Can you work these out from the model? Positions are in its coordinate system, mm. Face numbers are marked on the shaded views. A direction names the side the tool comes from. Give positions to 0.01 mm unless a question says otherwise; leave off trailing zeros. Order: outer loops, then holes, each group sorted by start corner. A loop starts at its lowest first (then second) coordinate and runs counter-clockwise, first axis right, second up.
Item 1: If I drill on line 1 along X through (y, z) = (15.75, 0); line 2 along Z through (x, y) = (-0.5, 4.5); line 3 along X through (y, z) = (9.5, -31), over which ranges is the centre line in solid material (lowest first)?
Item 2: Which directions (+Z, -Z, +X, -X, +Y, -Y) give clear straight access to the entire face, cutting with the end or side of a thin tool? Please do the marked faces 1, 2 and 3.
Item 3: I want a section at A-A, the plane x = 36. Write out the boundary of the cut face in (y, z).
Item 4: I want a section at B-B, the plane z = -36. Write out the boundary of the cut face in (x, y), then the cut area to 3 significant figures.
Item 5: I'm going to push flat-ended pins straight in: pin 1 Ø16 at (x, z) = (0, -11) entering from -Y; pin 2 Ø9 at (x, z) = (11, 0) entering from +Y; pin 3 Ø1.5 at (x, z) = (-8, 30) entering from -Y; pin 4 Ø4 at (y, z) = (2, -4) entering from -X. Where does each tip first touch, or does it pass through?
Item 6: If we mould it in two halves opening along X, with no side actions, what happens to the marked faces 4, 5 and 6? For each: +X half, -X half, draft (parallel to the pull), parting line (faces both ways), or undercut.
Item 7: I want a section at D-D, the plane z = 31. Write out the boundary of the cut face in (x, y).
Item 8: I want a section at C-C, the plane y = 15.75. Count the separate pieces of the cut face and the enclosed holes in it, then the cut area to 3 significant figures.
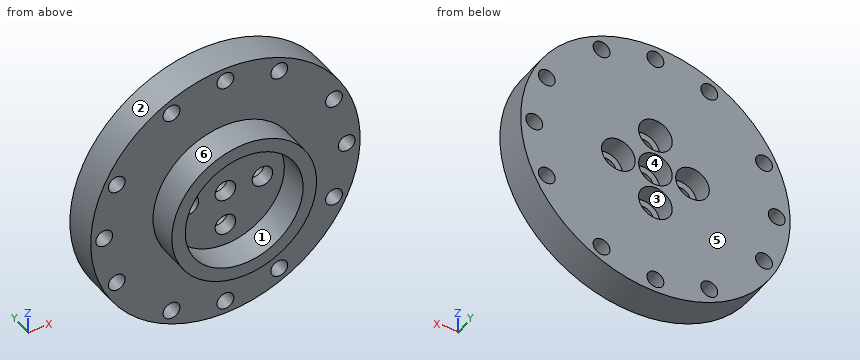
```python
from build123d import *

# Parameters (mm, degrees)
SKETCH1_R           = 21.5
SKETCH1_R_2         = 17.5
BOSS_EXTRUDE1_DEPTH = 9
SKETCH3_R           = 40
SKETCH3_R_2         = 3.05
SKETCH3_R_3         = 2.5
SKETCH3_R_4         = 2.496925047
SKETCH3_R_5         = 2.499529996
SKETCH3_R_6         = 2.502831222
SKETCH3_R_7         = 2.503585157
BOSS_EXTRUDE2_DEPTH = 10
CUT_EXTRUDE1_START  = -6
SKETCH6_R           = 5
SKETCH6_R_2         = 3.05
CUT_EXTRUDE1_DEPTH  = 6


with BuildPart() as part:
    # Sketch1 → Boss-Extrude1 (new body)
    with BuildSketch(Plane(origin=(0, 0, 0), x_dir=(1, 0, 0), z_dir=(0, 1, 0))):
        with Locations(Location((0, 0, 0), (0, 0, 270))):
            Circle(SKETCH1_R)
        with Locations(Location((0, 0, 0), (0, 0, 270))):
            Circle(SKETCH1_R_2, mode=Mode.SUBTRACT)
    extrude(amount=BOSS_EXTRUDE1_DEPTH)

    # Sketch3 → Boss-Extrude2 (add)
    with BuildSketch(Plane(origin=(0, 9, 0), x_dir=(1, 0, 0), z_dir=(0, 1, 0))):
        with Locations(Location((0, 0, 0), (0, 0, 270))):
            Circle(SKETCH3_R)
        with Locations(Location((0, 0, 0), (0, 0, 270))):
            Circle(SKETCH3_R_2, mode=Mode.SUBTRACT)
        with Locations(Location((-11, 0, 0), (0, 0, 270))):
            Circle(SKETCH3_R_2, mode=Mode.SUBTRACT)
        with Locations(Location((0, -11, 0), (0, 0, 270))):
            Circle(SKETCH3_R_2, mode=Mode.SUBTRACT)
        with Locations(Location((11, 0, 0), (0, 0, 270))):
            Circle(SKETCH3_R_2, mode=Mode.SUBTRACT)
        with Locations(Location((0, 11, 0), (0, 0, 270))):
            Circle(SKETCH3_R_2, mode=Mode.SUBTRACT)
        with Locations(Location((0, 36, 0), (0, 0, 270))):
            Circle(SKETCH3_R_3, mode=Mode.SUBTRACT)
        with Locations(Location((-32.251083055, 15.995863271, 0), (0, 0, 270))):
            Circle(SKETCH3_R_4, mode=Mode.SUBTRACT)
        with Locations(Location((-32.251083055, -15.995863271, 0), (0, 0, 270))):
            Circle(SKETCH3_R_5, mode=Mode.SUBTRACT)
        with Locations(Location((0, -36, 0), (0, 0, 270))):
            Circle(SKETCH3_R_3, mode=Mode.SUBTRACT)
        with Locations(Location((36, 0, 0), (0, 0, 270))):
            Circle(SKETCH3_R_3, mode=Mode.SUBTRACT)
        with Locations(Location((32.251083055, 15.995863271, 0), (0, 0, 270))):
            Circle(SKETCH3_R_6, mode=Mode.SUBTRACT)
        with Locations(Location((32.251083055, -15.995863271, 0), (0, 0, 270))):
            Circle(SKETCH3_R_3, mode=Mode.SUBTRACT)
        with Locations(Location((-16, 32.253585157, 0), (0, 0, 270))):
            Circle(SKETCH3_R_7, mode=Mode.SUBTRACT)
        with Locations(Location((16, 32.253585157, 0), (0, 0, 270))):
            Circle(SKETCH3_R_7, mode=Mode.SUBTRACT)
        with Locations(Location((-16, -32.25, 0), (0, 0, 270))):
            Circle(SKETCH3_R_3, mode=Mode.SUBTRACT)
        with Locations(Location((16, -32.25, 0), (0, 0, 270))):
            Circle(SKETCH3_R_3, mode=Mode.SUBTRACT)
        with Locations(Location((-36, 0, 0), (0, 0, 270))):
            Circle(SKETCH3_R_3, mode=Mode.SUBTRACT)
    extrude(amount=BOSS_EXTRUDE2_DEPTH)

    # Sketch6 → Cut-Extrude1 (cut)
    # profile 1 of 5: a face of its own
    with BuildSketch(Plane(origin=(0, 19, 0), x_dir=(1, 0, 0), z_dir=(0, 1, 0)).offset(CUT_EXTRUDE1_START)):
        with Locations(Location((0, 11, 0), (0, 0, 270))):
            Circle(SKETCH6_R)
        with Locations(Location((0, 11, 0), (0, 0, 270))):
            Circle(SKETCH6_R_2, mode=Mode.SUBTRACT)
    # profile 2 of 5: a face of its own
    with BuildSketch(Plane(origin=(0, 19, 0), x_dir=(1, 0, 0), z_dir=(0, 1, 0)).offset(CUT_EXTRUDE1_START)):
        with Locations(Location((-11, 0, 0), (0, 0, 270))):
            Circle(SKETCH6_R)
        with Locations(Location((-11, 0, 0), (0, 0, 270))):
            Circle(SKETCH6_R_2, mode=Mode.SUBTRACT)
    # profile 3 of 5: a face of its own
    with BuildSketch(Plane(origin=(0, 19, 0), x_dir=(1, 0, 0), z_dir=(0, 1, 0)).offset(CUT_EXTRUDE1_START)):
        with Locations(Location((0, 0, 0), (0, 0, 270))):
            Circle(SKETCH6_R)
        with Locations(Location((0, 0, 0), (0, 0, 270))):
            Circle(SKETCH6_R_2, mode=Mode.SUBTRACT)
    # profile 4 of 5: a face of its own
    with BuildSketch(Plane(origin=(0, 19, 0), x_dir=(1, 0, 0), z_dir=(0, 1, 0)).offset(CUT_EXTRUDE1_START)):
        with Locations(Location((11, 0, 0), (0, 0, 270))):
            Circle(SKETCH6_R)
        with Locations(Location((11, 0, 0), (0, 0, 270))):
            Circle(SKETCH6_R_2, mode=Mode.SUBTRACT)
    # profile 5 of 5: a face of its own
    with BuildSketch(Plane(origin=(0, 19, 0), x_dir=(1, 0, 0), z_dir=(0, 1, 0)).offset(CUT_EXTRUDE1_START)):
        with Locations(Location((0, -11, 0), (0, 0, 270))):
            Circle(SKETCH6_R)
        with Locations(Location((0, -11, 0), (0, 0, 270))):
            Circle(SKETCH6_R_2, mode=Mode.SUBTRACT)
    extrude(amount=CUT_EXTRUDE1_DEPTH, mode=Mode.SUBTRACT)


solid = part.part
```
Results list:
1. line 1: x = -40 to -38.5, -33.5 to -16, -6 to -5, 5 to 6, 16 to 33.5, 38.5 to 40
1. line 2: z = -21.49 to -17.49, 17.49 to 21.49
1. line 3: x = -25.28 to -18.17, -13.83 to 13.83, 18.17 to 25.28
2. face 1: -Y
2. face 2: +Y, -Y
2. face 3: +Y
3. outline: (9, -17.44) - (19, -17.44) - (19, -2.5) - (9, -2.5) - close; (9, 2.5) - (19, 2.5) - (19, 17.44) - (9, 17.44) - close
4. outline: (-17.44, 9) - (-2.5, 9) - (-2.5, 19) - (-17.44, 19) - close; (2.5, 9) - (17.44, 9) - (17.44, 19) - (2.5, 19) - close
4. area: 299 mm2
5. pin 1: stops at y = 0
5. pin 2: stops at y = 13
5. pin 3: stops at y = 9
5. pin 4: stops at x = -21.41
6. face 4: undercut
6. face 5: draft
6. face 6: parting line
7. outline: (-25.28, 9) - (-18.17, 9) - (-18.17, 19) - (-25.28, 19) - close; (-13.83, 9) - (13.83, 9) - (13.83, 19) - (-13.83, 19) - close; (18.17, 9) - (25.28, 9) - (25.28, 19) - (18.17, 19) - close
8. separate pieces: 1
8. enclosed holes: 17
8. area: 4,400 mm2
